Work out the finished part from the listing and answer in its coordinate system (mm). Coordinates: 2 decimals unless noted, no trailing zeros. Order: outer loops, then holes, each group sorted by start corner. A loop starts at its lowest first (then second) coordinate and runs counter-clockwise, first axis right, second up. Notation, with made-up numbers: (-32, 57.5) - (0, 57.5) arc R11 ccw to (0, 70.5) - close; hole circle Ø2 at (62, 50.25). An arc over 180 degrees is marked (long way). Use CSV: the item, a comma, the result in double quotes. Start each with the question number.
from build123d import *

# Parameters (mm, degrees)
F0_W     = 304.8
F0_H     = 304.8
F0_R     = 2.778125
F0_R_2   = 6.35
F0_R_3   = 2.667
F0_R_4   = 16.256
F1_DEPTH = 3.175


with BuildPart() as f1:
    # F0 (on Top) → F1 (new body)
    with BuildSketch(Plane.XY):
        with Locations((0, 50.8)):
            Rectangle(F0_W, F0_H)
        with Locations((-78.496965, -26.599268)):
            Circle(F0_R, mode=Mode.SUBTRACT)
        with Locations((-27.78125, -55.88)):
            Circle(F0_R, mode=Mode.SUBTRACT)
        with Locations((-131.7625, -25.4)):
            Circle(F0_R_2, mode=Mode.SUBTRACT)
        with Locations((-106.278215, 21.519268)):
            Circle(F0_R, mode=Mode.SUBTRACT)
        with Locations((-15.913014, -15.913014)):
            Circle(F0_R_3, mode=Mode.SUBTRACT)
        with Locations((-15.913014, 15.913014)):
            Circle(F0_R_3, mode=Mode.SUBTRACT)
        with Locations((27.78125, -55.88)):
            Circle(F0_R, mode=Mode.SUBTRACT)
        with Locations((78.496965, -26.599268)):
            Circle(F0_R, mode=Mode.SUBTRACT)
        with Locations((15.913014, -15.913014)):
            Circle(F0_R_3, mode=Mode.SUBTRACT)
        Circle(F0_R_4, mode=Mode.SUBTRACT)
        with Locations((15.913014, 15.913014)):
            Circle(F0_R_3, mode=Mode.SUBTRACT)
        with Locations((131.7625, -25.4)):
            Circle(F0_R_2, mode=Mode.SUBTRACT)
        with Locations((106.278215, 21.519268)):
            Circle(F0_R, mode=Mode.SUBTRACT)
        with Locations((-106.278215, 80.080732)):
            Circle(F0_R, mode=Mode.SUBTRACT)
        with Locations((-131.7625, 127)):
            Circle(F0_R_2, mode=Mode.SUBTRACT)
        with Locations((-78.496965, 128.199268)):
            Circle(F0_R, mode=Mode.SUBTRACT)
        with Locations((-27.78125, 157.48)):
            Circle(F0_R, mode=Mode.SUBTRACT)
        with Locations((0, 50.8)):
            Circle(F0_R_2, mode=Mode.SUBTRACT)
        with Locations((106.278215, 80.080732)):
            Circle(F0_R, mode=Mode.SUBTRACT)
        with Locations((27.78125, 157.48)):
            Circle(F0_R, mode=Mode.SUBTRACT)
        with Locations((78.496965, 128.199268)):
            Circle(F0_R, mode=Mode.SUBTRACT)
        with Locations((131.7625, 127)):
            Circle(F0_R_2, mode=Mode.SUBTRACT)
    extrude(amount=F1_DEPTH)


solid = f1.part
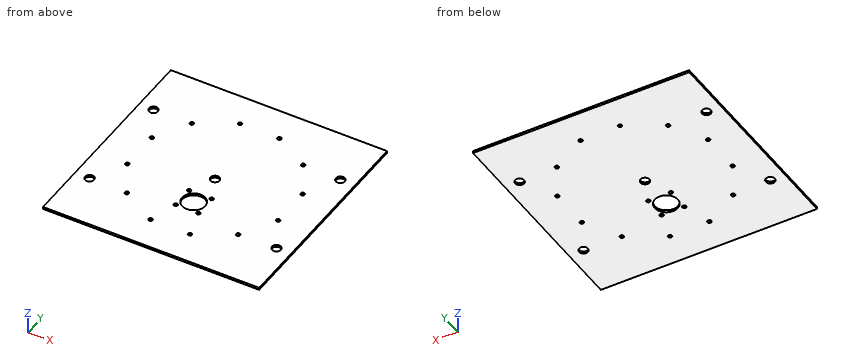
1) The part is cut by section D-D on z = 1.8. State how many separate pieces and enclosed holes the cut face has, plus the area to 3 significant figures.
2) The part is cut by section C-C on y = 0. Determine the outline of the cut face in (x, z) (3 decimals), plus the area to 3 significant figures.
3) Straight lines are drawn through the part: line 1 (X direction, y = 157.48, z = 0.8); line 2 (Y direction, x = 17, z = 1.75); line 3 (Y direction, x = -107, z = 0.9). For each, find the intervals that lie inside material, in ascending order. Write a range as [from, to].
4) The part is cut by section B-B on x = 0. Determine the outline of the cut face in (y, z) (3 decimals), plus the area to 3 significant figures.
5) Flat-ended cylindrical pins translate along their axes: P1, Ø6.5, axis at x = 78.5, y = 128.2, coming from the -Z side; P2, Ø11.5, axis at x = 0, y = 50.8, coming from the +Z side. Find the tip coordinate at first contact, or state that the pin passes through.
6) The part is cut by section A-A on y = 50.8. Determine the outline of the cut face in (x, z) (3 decimals).
Answer key:
1,separate pieces,"1"
1,enclosed holes,"22"
1,area,"91,100 mm^2"
2,outline,"(-152.4, 0) - (-16.256, 0) - (-16.256, 3.175) - (-152.4, 3.175) - close; (16.256, 0) - (152.4, 0) - (152.4, 3.175) - (16.256, 3.175) - close"
2,area,"865 mm^2"
3,line 1,"[-152.4, -30.56], [-25, 25], [30.56, 152.4]"
3,line 2,"[-101.6, -18.35], [-13.48, 13.48], [18.35, 203.2]"
3,line 3,"[-101.6, 18.84], [24.2, 77.4], [82.76, 203.2]"
4,outline,"(-101.6, 0) - (-16.256, 0) - (-16.256, 3.175) - (-101.6, 3.175) - close; (16.256, 0) - (44.45, 0) - (44.45, 3.175) - (16.256, 3.175) - close; (57.15, 0) - (203.2, 0) - (203.2, 3.175) - (57.15, 3.175) - close"
4,area,"824 mm^2"
5,P1,"z = 0"
5,P2,"through"
6,outline,"(-152.4, 0) - (-6.35, 0) - (-6.35, 3.175) - (-152.4, 3.175) - close; (6.35, 0) - (152.4, 0) - (152.4, 3.175) - (6.35, 3.175) - close"
